Read the model definition and answer for the solid it produces. Units are mm, in the model's axes. Face numbers are marked on the shaded views. A direction names the side the tool comes from. Give positions to 0.01 mm unless a question says otherwise; leave off trailing zeros. Loops run counter-clockwise (first coordinate to the right, second up) from the corner with the lowest first, then second, coordinate; pieces in that order, holes last. Notation, with made-up numbers: (48.5, -18) - (86.5, -18) arc R29 ccw to (86.5, 12) - close; hole circle Ø1 at (-2, 32.25). An arc over 180 degrees is marked (long way). Use a Markdown table: item, result. Add a question column.
Item 1: Which of the six approach directions +Z, -Z, +X, -X, +Y, -Y give full straight-line access (tool end or side, diameter ignored) to the marked faces 5, 6, 7, 8 and 9?
Item 2: For a pull along Z with two mould halves and no side action, classify the marked faces 1, 2, 3 and 4 as +Z half, -Z half, draft (parallel to the pull), parting line (faces both ways), or undercut.
Item 3: A cutting plane is placed at B-B (z = 14). Determine the outline of the cut face in (x, y), plus the area to 3 significant figures.
Item 4: A cutting plane is placed at A-A (y = 83). Determine the outline of the cut face in (x, z), plus the area to 3 significant figures.
Item 5: Each of these flat-tipped pins is pushed along its axis until it touches: P1, Ø21, axis at y = -207, z = 109, coming from the +X side; P2, Ø16, axis at y = -411.5, z = 60, coming from the -X side; P3, Ø3.5, axis at x = 63.5, y = -245, coming from the +Z side; P4, Ø10, axis at x = 789, y = -421, coming from the -Z side. Where does it stop, or does it pass through?
Item 6: Consider probe 1 along X at (y, z) = (88, -6.5); probe 2 along Y at (x, z) = (111.5, 497); probe 3 along Z at (x, y) = (714, 66.5). Determine where each line is inside the solid, lowest interval first. Write a range as [from, to].
Item 7: A cutting plane is placed at D-D (y = 183). Determine the outline of the cut face in (x, z).
Item 8: A cutting plane is placed at C-C (x = 804). Determine the outline of the cut face in (y, z), plus the area to 3 significant figures.
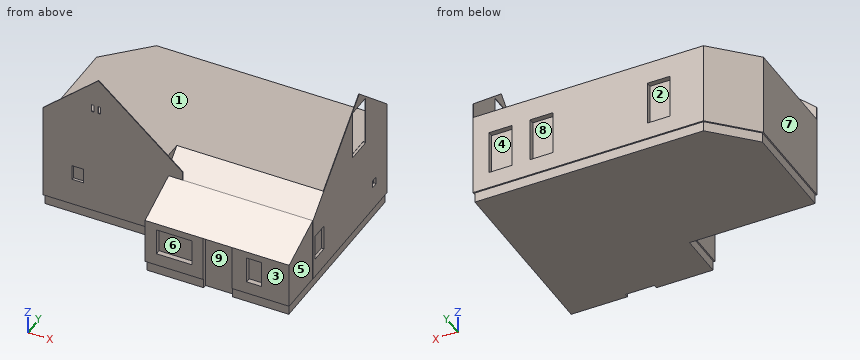
Solid Edge part; units mm, degrees
sketch "Sketch1" plane through (0, 0, 0) normal (0, 0, 1) x (1, 0, 0)
  line L0 (365.4075, -425.809) -> (935.4075, -425.809)
  line L1 (935.4075, -425.809) -> (935.4075, 319.191)
  line L2 (935.4075, 319.191) -> (25.4075, 319.191)
  line L3 (-130.5925, 163.191) -> (25.4075, 319.191)
  line L4 (-130.5925, -245.809) -> (-130.5925, 163.191)
  line L5 (365.4075, -245.809) -> (-130.5925, -245.809)
  line L6 (365.4075, -425.809) -> (365.4075, -245.809)
  dimension "D1" = 130.5925
  dimension "D2" = 365.4075
  dimension "D3" = 365.4075
  dimension "D4" = 365.4075
  dimension "D5" = 935.4075
  dimension "D6" = 935.4075
  dimension "D7" = 130.5925
extrude "Protrusion1" add sketch "Sketch1" along normal blind 330
sketch "Sketch2" plane through (365.4075, -335.809, 165) normal (-1, 0, 0) x (0, -1, 0)
  line L0 (90, 15) -> (-90, 90.5957)
  line L1 (-90, 90.5957) -> (-90, 165)
  line L2 (-90, 165) -> (90, 165)
  line L3 (90, 165) -> (90, 15)
extrude "Cutout1" cut sketch "Sketch2" against normal blind 730
sketch "Sketch3" plane through (935.4075, -53.309, 165) normal (1, 0, 0) x (0, 1, 0)
  line L0 (372.5, 90.5957) -> (372.5, 224.8613)
  line L1 (372.5, 224.8613) -> (160.7577, 410.5213)
  line L2 (-192.5, 90.5957) -> (160.7577, 410.5213)
  line L3 (-192.5, 90.5957) -> (372.5, 90.5957)
extrude "Protrusion2" add sketch "Sketch3" against normal blind 2
sketch "Sketch4" plane through (935.4075, -53.309, 261.575) normal (1, 0, 0) x (0, 1, 0)
  line L0 (-192.5, -5.9793) -> (-110.3437, 68.425)
  line L1 (-110.3437, 68.425) -> (-192.5, 68.425)
  line L2 (-192.5, 68.425) -> (-192.5, -5.9793)
extrude "ExtrudedCutout_40" cut sketch "Sketch4" against normal blind 580
sketch "Sketch5" plane through (117.4075, -245.809, 165) normal (0, -1, 0) x (1, 0, 0)
  line L0 (303.4101, 90.5957) -> (303.4101, 125)
  line L1 (303.4101, 125) -> (-29.1781, 411.2644)
  line L2 (-29.1781, 411.2644) -> (-248, 217.6121)
  line L3 (-248, 217.6121) -> (-248, 90.5957)
  line L4 (-248, 90.5957) -> (303.4101, 90.5957)
extrude "Protrusion3" add sketch "Sketch5" against normal blind 3
sketch "Sketch6" plane through (402.4075, -53.309, 0) normal (0, 0, -1) x (1, 0, 0)
  line L0 (528, 367.5) -> (528, -367.5)
  line L1 (528, -367.5) -> (-374.9289, -367.5)
  line L2 (-374.9289, -367.5) -> (-528, -214.4289)
  line L3 (-528, -214.4289) -> (-528, 187.5)
  line L4 (-528, 187.5) -> (-32, 187.5)
  line L5 (-32, 187.5) -> (-32, 367.5)
  line L6 (-32, 367.5) -> (528, 367.5)
extrude "ExtrudedProtrusion_65" add sketch "Sketch6" along normal blind 40
sketch "Sketch7" plane through (935.4075, -53.309, 261.575) normal (1, 0, 0) x (0, 1, 0)
  line L0 (110.0542, 67.3904) -> (210.0542, 67.3904)
  line L1 (210.0542, 67.3904) -> (210.0542, 263.8741)
  line L2 (210.0542, 263.8741) -> (110.0542, 263.8741)
  line L3 (110.0542, 263.8741) -> (110.0542, 67.3904)
  line L4 (-178.8496, -185.6242) -> (-108.8496, -185.6242)
  line L5 (-108.8496, -185.6242) -> (-108.8496, -85.6242)
  line L6 (-108.8496, -85.6242) -> (-178.8496, -85.6242)
  line L7 (-178.8496, -85.6242) -> (-178.8496, -185.6242)
  line L8 (260.1448, -166.6553) -> (290.1448, -166.6553)
  line L9 (290.1448, -166.6553) -> (290.1448, -136.6553)
  line L10 (290.1448, -136.6553) -> (260.1448, -136.6553)
  line L11 (260.1448, -136.6553) -> (260.1448, -166.6553)
extrude "Cutout2" cut sketch "Sketch7" against normal blind 10
sketch "Sketch8" plane through (650.4075, -425.809, 90) normal (0, -1, 0) x (1, 0, 0)
  line L0 (-56.5636, -130) -> (58.4364, -130)
  line L1 (58.4364, -130) -> (58.4364, 90)
  line L2 (58.4364, 90) -> (-56.5636, 90)
  line L3 (-56.5636, 90) -> (-56.5636, -130)
  line L4 (115.641, -40.8515) -> (175.641, -40.8515)
  line L5 (175.641, -40.8515) -> (175.641, 64.1485)
  line L6 (175.641, 64.1485) -> (115.641, 64.1485)
  line L7 (115.641, 64.1485) -> (115.641, -40.8515)
  line L8 (-240.0809, -40.8515) -> (-100.0809, -40.8515)
  line L9 (-100.0809, -40.8515) -> (-100.0809, 64.1485)
  line L10 (-100.0809, 64.1485) -> (-240.0809, 64.1485)
  line L11 (-240.0809, 64.1485) -> (-240.0809, -40.8515)
extrude "ExtrudedCutout_42" cut sketch "Sketch8" against normal blind 20
sketch "Sketch9" plane through (145.1125, -245.809, 288.1322) normal (0, -1, 0) x (1, 0, 0)
  line L0 (-161.1882, -180.5905) -> (-116.1882, -180.5905)
  line L1 (-116.1882, -180.5905) -> (-116.1882, -120.5905)
  line L2 (-116.1882, -120.5905) -> (-161.1882, -120.5905)
  line L3 (-161.1882, -120.5905) -> (-161.1882, -180.5905)
  line L4 (-58.0225, 144.6205) -> (-48.0225, 144.6205)
  line L5 (-48.0225, 144.6205) -> (-48.0225, 174.6205)
  line L6 (-48.0225, 174.6205) -> (-58.0225, 174.6205)
  line L7 (-58.0225, 174.6205) -> (-58.0225, 144.6205)
  line L8 (-84.855, 144.6205) -> (-74.855, 144.6205)
  line L9 (-74.855, 144.6205) -> (-74.855, 174.6205)
  line L10 (-74.855, 174.6205) -> (-84.855, 174.6205)
  line L11 (-84.855, 174.6205) -> (-84.855, 144.6205)
extrude "Cutout3" cut sketch "Sketch9" against normal blind 10
sketch "Sketch10" plane through (480.4075, 319.191, 194.9306) normal (0, 1, 0) x (-1, 0, 0)
  line L0 (-391.7685, -128.2335) -> (-301.7685, -128.2335)
  line L1 (-301.7685, -128.2335) -> (-301.7685, 46.7665)
  line L2 (-301.7685, 46.7665) -> (-391.7685, 46.7665)
  line L3 (-391.7685, 46.7665) -> (-391.7685, -128.2335)
  line L4 (-229.3403, -128.2335) -> (-139.3403, -128.2335)
  line L5 (-139.3403, -128.2335) -> (-139.3403, 46.7665)
  line L6 (-139.3403, 46.7665) -> (-229.3403, 46.7665)
  line L7 (-229.3403, 46.7665) -> (-229.3403, -128.2335)
  line L8 (233.108, -128.2335) -> (323.108, -128.2335)
  line L9 (323.108, -128.2335) -> (323.108, 46.7665)
  line L10 (323.108, 46.7665) -> (233.108, 46.7665)
  line L11 (233.108, 46.7665) -> (233.108, -128.2335)
extrude "Cutout4" cut sketch "Sketch10" against normal blind 20
sketch "Sketch11" plane through (935.4075, -53.309, 287.7607) normal (1, 0, 0) x (0, 1, 0)
  line L0 (-372.5, -107.7607) -> (-192.5, -32.165)
  line L1 (-192.5, -32.165) -> (-192.5, -287.7607)
  line L2 (-192.5, -287.7607) -> (-372.5, -287.7607)
  line L3 (-372.5, -287.7607) -> (-372.5, -107.7607)
extrude "Cutout5" cut sketch "Sketch11" against normal blind 1
Geometry says:
| question | item | result |
|---|---|---|
| 1 | face 5 | +Z, -Z, +X, -Y |
| 1 | face 6 | -Y |
| 1 | face 7 | +Z, -Z, -X, +Y, -Y |
| 1 | face 8 | +Y |
| 1 | face 9 | -Z, -Y |
| 2 | face 1 | +Z half |
| 2 | face 2 | undercut |
| 2 | face 3 | draft |
| 2 | face 4 | undercut |
| 3 | outline | (-130.59, -245.81) - (365.41, -245.81) - (365.41, -425.81) - (593.84, -425.81) - (593.84, -405.81) - (708.84, -405.81) - (708.84, -425.81) - (934.41, -425.81) - (934.41, -245.81) - (935.41, -245.81) - (935.41, 319.19) - (25.41, 319.19) - (-130.59, 163.19) - close |
| 3 | area | 690,000 mm² |
| 4 | outline | (-130.59, 0) - (-125.59, 0) - (-125.59, -40) - (930.41, -40) - (930.41, 0) - (935.41, 0) - (935.41, 328.97) - (925.41, 328.97) - (925.41, 330) - (-130.59, 330) - close; (933.41, 525.45) - (935.41, 525.45) - (935.41, 553.38) - (933.41, 553.38) - close |
| 4 | area | 394,000 mm² |
| 5 | P1 | x = 925.41 |
| 5 | P2 | x = 365.41 |
| 5 | P3 | z = 555.93 |
| 5 | P4 | z = -40 |
| 6 | probe 1 | [-125.59, 930.41] |
| 6 | probe 2 | [-245.81, -242.81] |
| 6 | probe 3 | [-40, 330] |
| 7 | outline | (-110.78, 0) - (-103.71, 0) - (-103.71, -40) - (930.41, -40) - (930.41, 0) - (935.41, 0) - (935.41, 509.28) - (933.41, 509.28) - (933.41, 330) - (-110.78, 330) - close |
| 8 | outline | (-425.81, 0) - (-420.81, 0) - (-420.81, -40) - (314.19, -40) - (314.19, 0) - (319.19, 0) - (319.19, 66.7) - (299.19, 66.7) - (299.19, 241.7) - (319.19, 241.7) - (319.19, 330) - (-163.65, 330) - (-245.81, 255.6) - (-425.81, 180) - (-425.81, 154.15) - (-405.81, 154.15) - (-405.81, 49.15) - (-425.81, 49.15) - close |
| 8 | area | 246,000 mm² |
